Geometry: final body of the model. Coordinates: model frame, mm. Face numbers are marked on the shaded views. A direction names the side the tool comes from. Coordinates: 2 decimals unless noted, no trailing zeros. Order: outer loops, then holes, each group sorted by start corner. A loop starts at its lowest first (then second) coordinate and runs counter-clockwise, first axis right, second up. Notation, with made-up numbers: (26.5, -20) -> (47.5, -20) arc R17 cw to (47.5, -16) -> close; hole circle Ø6 at (44.25, -16). An arc over 180 degrees is marked (long way). Answer in a Markdown table with one row per item. Add a question column.
1) Ray query, line 1 (X direction, y = -65, z = 0); line 2 (X direction, y = 47.5, z = 9); line 3 (Z direction, x = -52, y = -26). Return the intervals inside material, ascending. Write a range as from..to.
2) Contact query for flat-ended pins moving along their axis: P1, Ø8, axis at x = 45.5, z = 2, coming from the +Y side; P2, Ø6, axis at x = -4.5, z = 4, coming from the +Y side; P3, Ø6, axis at y = 63.5, z = 11.5, coming from the -X side. Output: stop coordinate, or through.
3) Section query A-A on x = 0. Return the cut outline in (y, z).
4) Section query C-C on z = 13. Return the cut outline in (x, y).
5) Set-up query: the marked faces 1 and 2. Return all of +Z, -Z, +X, -X, +Y, -Y with unobstructed straight access to the full face (end or side cutting, diameter ignored); none if empty.
6) Section query D-D on x = -20. Return the cut outline in (y, z).
7) Section query B-B on z = -1.5. Return the cut outline in (x, y), then the cut area to 3 significant figures.
8) Pull-direction query (Z, two-part tool) for the marked faces 3, 4 and 5; classes: +Z half, -Z half, draft (parallel to the pull), parting line (faces both ways), or undercut.
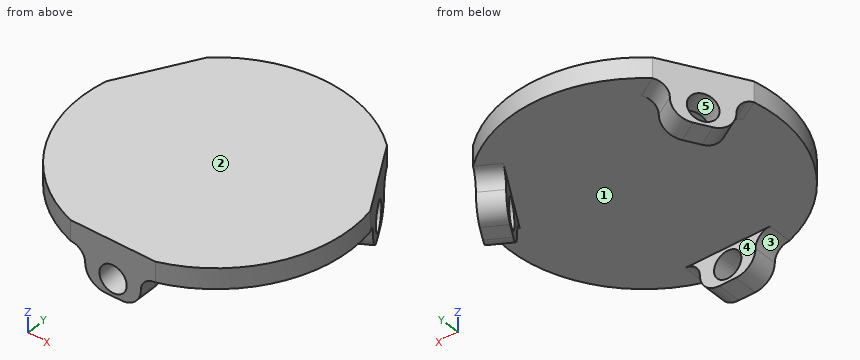
```python
from build123d import *

# Parameters (mm, degrees)
SKETCH2_R                   = 79
BOSS_EXTRUDE1_DEPTH         = 12
SKETCH2_3_W                 = 49.638694584
SKETCH2_3_H                 = 14
CUT_EXTRUDE1_DEPTH          = 113.365475125
SKETCH2_4_W                 = 49.638694584
SKETCH2_4_H                 = 14
BOSS_EXTRUDE2_DEPTH         = 20
SKETCH3_R                   = 8
CUT_EXTRUDE2_DEPTH          = 175.232603149
CIRPATTERN1_COUNT           = 3
CIRPATTERN1_COPY_1_SKETCH_R = 8
CIRPATTERN1_COPY_1_DEPTH    = 175.232603149
CIRPATTERN1_COPY_2_SKETCH_R = 8
CIRPATTERN1_COPY_2_DEPTH    = 175.232603149


with BuildPart() as part:
    # Sketch2 → Boss-Extrude1 (new body)
    with BuildSketch(Plane.XY):
        Circle(SKETCH2_R)
    extrude(amount=BOSS_EXTRUDE1_DEPTH)

    # Sketch2<3> → Cut-Extrude1 (cut, symmetric)
    with BuildSketch(Plane.XY):
        with Locations((0, -82)):
            Rectangle(SKETCH2_3_W, SKETCH2_3_H)
    cut_extrude1 = extrude(amount=CUT_EXTRUDE1_DEPTH, both=True, mode=Mode.SUBTRACT)

    # Sketch2<4> → Boss-Extrude2 (add)
    with BuildSketch(Plane.XY):
        with Locations((0, -68)):
            Rectangle(SKETCH2_4_W, SKETCH2_4_H)
    boss_extrude2 = extrude(amount=-BOSS_EXTRUDE2_DEPTH)

    # Sketch3 → Cut-Extrude2 (cut, symmetric)
    with BuildSketch(Plane.XZ.offset(75)):
        with Locations(Location((0, -10, 0), (0, 0, 270))):
            Circle(SKETCH3_R)
        with BuildLine():
            Line((-24.819347292, 0), (-24.819347292, -20))
            Line((-24.819347292, -20), (-4.819347292, -20))
            ThreePointArc((-4.819347292, -20), (-12.938662868, -16.636869371), (-16.301793497, -8.517553795))
            ThreePointArc((-16.301793497, -8.517553795), (-18.796527244, -2.494733747), (-24.819347292, 0))
        make_face()
    cut_extrude2 = extrude(amount=CUT_EXTRUDE2_DEPTH, both=True, mode=Mode.SUBTRACT)

    # Mirror1: Cut-Extrude2 across plane
    add(cut_extrude2.mirror(Plane(origin=(0, 0, 0), x_dir=(0, 0, 1), z_dir=(1, 0, 0))), mode=Mode.SUBTRACT)

    # CirPattern1: Cut-Extrude1, Boss-Extrude2, Cut-Extrude2 ×3 about axis
    cirpattern1_axis = Axis((0, 0, 0), (0, 0, 1))
    add([cut_extrude1.rotate(cirpattern1_axis, i * 360 / CIRPATTERN1_COUNT) for i in range(1, CIRPATTERN1_COUNT)], mode=Mode.SUBTRACT)
    add([boss_extrude2.rotate(cirpattern1_axis, i * 360 / CIRPATTERN1_COUNT) for i in range(1, CIRPATTERN1_COUNT)])
    add([cut_extrude2.rotate(cirpattern1_axis, i * 360 / CIRPATTERN1_COUNT) for i in range(1, CIRPATTERN1_COUNT)], mode=Mode.SUBTRACT)

    # CirPattern1 copy 1 sketch → CirPattern1 copy 1 (cut, symmetric)
    with BuildSketch(Plane(origin=(64.951905284, 37.5, 0), x_dir=(0.4999999999999998, -0.8660254037844387, 0), z_dir=(0.8660254037844387, 0.4999999999999998, 0))):
        with Locations((0, 10)):
            Circle(CIRPATTERN1_COPY_1_SKETCH_R)
        with BuildLine():
            Line((-24.819347292, 0), (-24.819347292, 20))
            Line((-24.819347292, 20), (-4.819347292, 20))
            ThreePointArc((-4.819347292, 20), (-12.938662868, 16.636869371), (-16.301793497, 8.517553795))
            ThreePointArc((-16.301793497, 8.517553795), (-18.796527244, 2.494733747), (-24.819347292, 0))
        make_face()
    extrude(amount=CIRPATTERN1_COPY_1_DEPTH, both=True, mode=Mode.SUBTRACT)

    # CirPattern1 copy 2 sketch → CirPattern1 copy 2 (cut, symmetric)
    with BuildSketch(Plane(origin=(-64.951905284, 37.5, 0), x_dir=(0.5000000000000004, 0.8660254037844384, 0), z_dir=(-0.8660254037844384, 0.5000000000000004, 0))):
        with Locations((0, 10)):
            Circle(CIRPATTERN1_COPY_2_SKETCH_R)
        with BuildLine():
            Line((-24.819347292, 0), (-24.819347292, 20))
            Line((-24.819347292, 20), (-4.819347292, 20))
            ThreePointArc((-4.819347292, 20), (-12.938662868, 16.636869371), (-16.301793497, 8.517553795))
            ThreePointArc((-16.301793497, 8.517553795), (-18.796527244, 2.494733747), (-24.819347292, 0))
        make_face()
    extrude(amount=CIRPATTERN1_COPY_2_DEPTH, both=True, mode=Mode.SUBTRACT)


with BuildPart() as part_1:
    # Body-Move/Copy1: moved
    add(part.part.moved(Location((0, -5e-08, 10))))


solid = part_1.part
```
Result:
| question | item | result |
|---|---|---|
| 1 | line 1 | -16.21..-8, 8..16.21 |
| 1 | line 2 | -59.18..-43.01, 43.01..59.18 |
| 1 | line 3 | 10..22 |
| 2 | P1 | y = 47.54 |
| 2 | P2 | y = -61 |
| 2 | P3 | x = -50.8 |
| 3 | outline | (-75, -10) -> (-61, -10) -> (-61, -8) -> (-75, -8) -> close; (-75, 8) -> (-61, 8) -> (-61, 10) -> (79, 10) -> (79, 22) -> (-75, 22) -> close |
| 4 | outline | (-77.36, 16.01) arc R79 ccw to (-24.82, -75) -> (24.82, -75) arc R79 ccw to (77.36, 16.01) -> (52.54, 58.99) arc R79 ccw to (-52.54, 58.99) -> close |
| 5 | face 1 | -Z |
| 5 | face 2 | +Z, +X, -X, +Y, -Y |
| 6 | outline | (-75, 8.51) -> (-61, 8.51) -> (-61, 10) -> (76.43, 10) -> (76.43, 22) -> (-75, 22) -> close |
| 7 | outline | (-72.91, 23.72) -> (-60.78, 16.72) -> (-56.76, 23.69) -> (-68.88, 30.69) -> close; (-61.02, 44.31) -> (-48.9, 37.31) -> (-44.87, 44.28) -> (-57, 51.28) -> close; (-15.91, -75) -> (-7.86, -75) -> (-7.86, -61) -> (-15.91, -61) -> close; (7.86, -75) -> (15.91, -75) -> (15.91, -61) -> (7.86, -61) -> close; (44.87, 44.28) -> (48.9, 37.31) -> (61.02, 44.31) -> (57, 51.28) -> close; (56.76, 23.69) -> (60.78, 16.72) -> (72.91, 23.72) -> (68.88, 30.69) -> close |
| 7 | area | 676 mm2 |
| 8 | face 3 | -Z half |
| 8 | face 4 | draft |
| 8 | face 5 | undercut |
